```python
from build123d import *

# Parameters (mm, degrees)
SKETCH2_W                                            = 184.15
SKETCH2_H                                            = 190.5
BOSS_EXTRUDE1_DEPTH                                  = 50.8
SHELL1_T                                             = -5.08
CSK_FOR_M6_HEX_SOCKET_COUNTERSUNK_CAP_SC_D           = 6.6
CSK_FOR_M6_HEX_SOCKET_COUNTERSUNK_CAP_SC_DEPTH       = 11.733159957
CSK_FOR_M6_HEX_SOCKET_COUNTERSUNK_CAP_SC_CSINK_D     = 13.44
CSK_FOR_M6_HEX_SOCKET_COUNTERSUNK_CAP_SC_CSINK_ANGLE = 90
CSK_FOR_M6_HEX_SOCKET_COUNTERSUNK_CAP_SC_TIP         = 1.982840043
FILLET1_R                                            = 2.54


with BuildPart() as part:
    # Sketch2 → Boss-Extrude1 (new body)
    with BuildSketch(Plane(origin=(0, 0, 0), x_dir=(1, 0, 0), z_dir=(0, 1, 0))):
        Rectangle(SKETCH2_W, SKETCH2_H)
    extrude(amount=-BOSS_EXTRUDE1_DEPTH)

    # Shell1
    shell1_openings = [part.faces().sort_by_distance(p)[0] for p in [
        (0, -50.8, 0),
    ]]
    offset(amount=SHELL1_T, openings=shell1_openings, kind=Kind.INTERSECTION)

    # Loft1: read off the stored shape, not the designer's step
    # Loft1: loft between two sections, ruled curve by curve
    loft1_from = [
        Edge.make_bspline([(68.241223487, -26.310119776, -101.6), (68.532768976, -26.616911457, -101.6), (68.863871753, -26.909333008, -101.6), (69.601572379, -27.439191099, -101.6), (70.008225028, -27.676441112, -101.6), (70.882099248, -28.069631586, -101.6), (71.349251098, -28.225355381, -101.6), (72.31767022, -28.435607084, -101.6), (72.818735502, -28.489985667, -101.6), (73.821125836, -28.489985667, -101.6), (74.322191118, -28.435607084, -101.6), (75.29061024, -28.225355381, -101.6), (75.757762089, -28.069631586, -101.6), (76.631636309, -27.676441112, -101.6), (77.038288959, -27.439191099, -101.6), (77.775989584, -26.909333008, -101.6), (78.107092362, -26.616911457, -101.6), (78.39863785, -26.310119776, -101.6)], [0, 0, 0, 0, 0.125, 0.125, 0.25, 0.25, 0.375, 0.375, 0.5, 0.5, 0.625, 0.625, 0.75, 0.75, 0.875, 0.875, 1, 1, 1, 1], 3),
        Edge.make_bspline([(78.39863785, -26.310119776, -101.6), (78.675694815, -26.018574288, -101.6), (78.937226358, -25.692808769, -101.6), (79.407739121, -24.977845102, -101.6), (79.616581189, -24.588623733, -101.6), (79.961046476, -23.760489668, -101.6), (80.096520237, -23.321639377, -101.6), (80.279103538, -22.416392759, -101.6), (80.326114413, -21.950142771, -101.6), (80.326114413, -21.017461075, -101.6), (80.279103538, -20.551211086, -101.6), (80.096520237, -19.645964468, -101.6), (79.961046476, -19.207114178, -101.6), (79.616581189, -18.378980112, -101.6), (79.407739121, -17.989758743, -101.6), (78.937226358, -17.274795077, -101.6), (78.675694815, -16.949029558, -101.6), (78.39863785, -16.657484069, -101.6)], [0, 0, 0, 0, 0.125, 0.125, 0.25, 0.25, 0.375, 0.375, 0.5, 0.5, 0.625, 0.625, 0.75, 0.75, 0.875, 0.875, 1, 1, 1, 1], 3),
        Edge.make_bspline([(68.241223487, -16.657484069, -101.6), (67.964166523, -16.949029558, -101.6), (67.70263498, -17.274795077, -101.6), (67.232122217, -17.989758743, -101.6), (67.023280149, -18.378980112, -101.6), (66.678814862, -19.207114178, -101.6), (66.543341101, -19.645964468, -101.6), (66.3607578, -20.551211086, -101.6), (66.313746925, -21.017461075, -101.6), (66.313746925, -21.950142771, -101.6), (66.3607578, -22.416392759, -101.6), (66.543341101, -23.321639377, -101.6), (66.678814862, -23.760489668, -101.6), (67.023280149, -24.588623733, -101.6), (67.232122217, -24.977845102, -101.6), (67.70263498, -25.692808769, -101.6), (67.964166523, -26.018574288, -101.6), (68.241223487, -26.310119776, -101.6)], [0, 0, 0, 0, 0.125, 0.125, 0.25, 0.25, 0.375, 0.375, 0.5, 0.5, 0.625, 0.625, 0.75, 0.75, 0.875, 0.875, 1, 1, 1, 1], 3),
        Edge.make_bspline([(78.39863785, -16.657484069, -101.6), (78.107092362, -16.350692388, -101.6), (77.775989584, -16.058270838, -101.6), (77.038288959, -15.528412746, -101.6), (76.631636309, -15.291162733, -101.6), (75.757762089, -14.89797226, -101.6), (75.29061024, -14.742248464, -101.6), (74.322191118, -14.531996762, -101.6), (73.821125836, -14.477618178, -101.6), (72.818735502, -14.477618178, -101.6), (72.31767022, -14.531996762, -101.6), (71.349251098, -14.742248464, -101.6), (70.882099248, -14.89797226, -101.6), (70.008225028, -15.291162733, -101.6), (69.601572379, -15.528412746, -101.6), (68.863871753, -16.058270838, -101.6), (68.532768976, -16.350692388, -101.6), (68.241223487, -16.657484069, -101.6)], [0, 0, 0, 0, 0.125, 0.125, 0.25, 0.25, 0.375, 0.375, 0.5, 0.5, 0.625, 0.625, 0.75, 0.75, 0.875, 0.875, 1, 1, 1, 1], 3),
    ]
    loft1_to = [
        Edge.make_bspline([(62.059516528, -35.333897225, -95.25), (63.205579438, -35.333897225, -95.25), (64.351642348, -35.333897225, -95.25), (66.643768167, -35.333897225, -95.25), (67.789831077, -35.333897225, -95.25), (70.081956897, -35.333897225, -95.25), (71.228019807, -35.333897225, -95.25), (73.520145626, -35.333897225, -95.25), (74.666208536, -35.333897225, -95.25), (76.958334356, -35.333897225, -95.25), (78.104397266, -35.333897225, -95.25), (80.396523085, -35.333897225, -95.25), (81.542585995, -35.333897225, -95.25), (83.834711815, -35.333897225, -95.25), (84.980774725, -35.333897225, -95.25), (87.272900544, -35.333897225, -95.25), (88.418963454, -35.333897225, -95.25), (89.565026364, -35.333897225, -95.25)], [0, 0, 0, 0, 0.125, 0.125, 0.25, 0.25, 0.375, 0.375, 0.5, 0.5, 0.625, 0.625, 0.75, 0.75, 0.875, 0.875, 1, 1, 1, 1], 3),
        Edge.make_bspline([(89.565026364, -35.333897225, -95.25), (89.565026364, -34.244788582, -95.25), (89.565026364, -33.15567994, -95.25), (89.565026364, -30.977462655, -95.25), (89.565026364, -29.888354013, -95.25), (89.565026364, -27.710136729, -95.25), (89.565026364, -26.621028086, -95.25), (89.565026364, -24.442810802, -95.25), (89.565026364, -23.353702159, -95.25), (89.565026364, -21.175484875, -95.25), (89.565026364, -20.086376233, -95.25), (89.565026364, -17.908158948, -95.25), (89.565026364, -16.819050306, -95.25), (89.565026364, -14.640833021, -95.25), (89.565026364, -13.551724379, -95.25), (89.565026364, -11.373507094, -95.25), (89.565026364, -10.284398452, -95.25), (89.565026364, -9.19528981, -95.25)], [0, 0, 0, 0, 0.125, 0.125, 0.25, 0.25, 0.375, 0.375, 0.5, 0.5, 0.625, 0.625, 0.75, 0.75, 0.875, 0.875, 1, 1, 1, 1], 3),
        Edge.make_bspline([(62.059516528, -9.19528981, -95.25), (62.059516528, -10.284398452, -95.25), (62.059516528, -11.373507094, -95.25), (62.059516528, -13.551724379, -95.25), (62.059516528, -14.640833021, -95.25), (62.059516528, -16.819050306, -95.25), (62.059516528, -17.908158948, -95.25), (62.059516528, -20.086376233, -95.25), (62.059516528, -21.175484875, -95.25), (62.059516528, -23.353702159, -95.25), (62.059516528, -24.442810802, -95.25), (62.059516528, -26.621028086, -95.25), (62.059516528, -27.710136729, -95.25), (62.059516528, -29.888354013, -95.25), (62.059516528, -30.977462655, -95.25), (62.059516528, -33.15567994, -95.25), (62.059516528, -34.244788582, -95.25), (62.059516528, -35.333897225, -95.25)], [0, 0, 0, 0, 0.125, 0.125, 0.25, 0.25, 0.375, 0.375, 0.5, 0.5, 0.625, 0.625, 0.75, 0.75, 0.875, 0.875, 1, 1, 1, 1], 3),
        Edge.make_bspline([(89.565026364, -9.19528981, -95.25), (88.418963454, -9.19528981, -95.25), (87.272900544, -9.19528981, -95.25), (84.980774725, -9.19528981, -95.25), (83.834711815, -9.19528981, -95.25), (81.542585995, -9.19528981, -95.25), (80.396523085, -9.19528981, -95.25), (78.104397266, -9.19528981, -95.25), (76.958334356, -9.19528981, -95.25), (74.666208536, -9.19528981, -95.25), (73.520145626, -9.19528981, -95.25), (71.228019807, -9.19528981, -95.25), (70.081956897, -9.19528981, -95.25), (67.789831077, -9.19528981, -95.25), (66.643768167, -9.19528981, -95.25), (64.351642348, -9.19528981, -95.25), (63.205579438, -9.19528981, -95.25), (62.059516528, -9.19528981, -95.25)], [0, 0, 0, 0, 0.125, 0.125, 0.25, 0.25, 0.375, 0.375, 0.5, 0.5, 0.625, 0.625, 0.75, 0.75, 0.875, 0.875, 1, 1, 1, 1], 3),
    ]
    loft1 = Solid(Shell([*[Face.make_surface_from_curves(loft1_from[k], loft1_to[k]) for k in range(4)], Face(Wire(loft1_from)), Face(Wire(loft1_to))]))
    add(loft1)

    # CSK for M6 Hex Socket Countersunk Cap Screw1
    with Locations(Plane(origin=(0, 0, -101.6), x_dir=(-1, 0, 0), z_dir=(0, 0, -1))):
        with Locations((-73.319930669, -21.483801923)):
            CounterSinkHole(CSK_FOR_M6_HEX_SOCKET_COUNTERSUNK_CAP_SC_D / 2, CSK_FOR_M6_HEX_SOCKET_COUNTERSUNK_CAP_SC_CSINK_D / 2, depth=CSK_FOR_M6_HEX_SOCKET_COUNTERSUNK_CAP_SC_DEPTH, counter_sink_angle=CSK_FOR_M6_HEX_SOCKET_COUNTERSUNK_CAP_SC_CSINK_ANGLE)
            with Locations((0, 0, -(CSK_FOR_M6_HEX_SOCKET_COUNTERSUNK_CAP_SC_DEPTH + CSK_FOR_M6_HEX_SOCKET_COUNTERSUNK_CAP_SC_TIP / 2))):  # 118° drill point
                Cone(0, CSK_FOR_M6_HEX_SOCKET_COUNTERSUNK_CAP_SC_D / 2, CSK_FOR_M6_HEX_SOCKET_COUNTERSUNK_CAP_SC_TIP, mode=Mode.SUBTRACT)

    # Fillet1
    fillet1_edges = [part.edges().sort_by_distance(p)[0] for p in [
        (0, 0, 95.25),
        (-92.075, 0, 0),
        (0, 0, -95.25),
        (92.075, 0, 0),
    ]]
    fillet(fillet1_edges, radius=FILLET1_R)


solid = part.part
```
Model file for the job. Use its own axes, mm. A direction names the side the tool comes from. Give positions to 0.01 mm unless a question says otherwise; leave off trailing zeros. Loops run counter-clockwise (first coordinate to the right, second up) from the corner with the lowest first, then second, coordinate; pieces in that order, holes last. Notation, with made-up numbers: (83, 58) -> (141, 58) arc R38 cw to (141, 96) -> close; hole circle Ø7 at (-36.75, -33.5). An arc over 180 degrees is marked (long way). Write each question's results on one line, items separated by ' | '.
(1) Tool access for faces 4 (the flat face through (-86.995, -28, 1)), 5 (the flat face through (-92.075, -26, 1)): list every direction of +Z, -Z, +X, -X, +Y, -Y with a clear straight run to the whole face (end or side of a thin tool).
Geometry results:
face 4: -Y | face 5: +Z, -Z, -X, +Y, -Y
(2) Cut at A-A on z = 26. List the corners of the cut face in (x, y) (3 decimals).
Geometry results:
outline: (-92.075, -50.8) -> (-86.995, -50.8) -> (-86.995, -5.08) -> (86.995, -5.08) -> (86.995, -50.8) -> (92.075, -50.8) -> (92.075, -2.54) arc R2.54 ccw to (89.535, 0) -> (-89.535, 0) arc R2.54 ccw to (-92.075, -2.54) -> close
(3) Cut at B-B on x = -73. List the corners of the cut face in (y, z), and give its area (3 significant figures).
Geometry results:
outline: (-50.8, -95.25) -> (-2.54, -95.25) arc R2.54 ccw to (0, -92.71) -> (0, 92.71) arc R2.54 ccw to (-2.54, 95.25) -> (-50.8, 95.25) -> (-50.8, 90.17) -> (-5.08, 90.17) -> (-5.08, -90.17) -> (-50.8, -90.17) -> close | area: 1,430 mm²
(4) Pull direction X, two halves, no side cores. Call faces 1 (the flat face through (92.075, -26, 1)), 2 (the flat face through (-1, -26, 95.25)), 3 (the cylindrical face through (76.468, -20.493, -94.119)): released by +X, released by -X, zero draft, split by the parting line, or undercut.
Geometry results:
face 1: released by +X | face 2: zero draft | face 3: undercut
(5) Probe line 1 along Z through (x, y) = (-61.5, -13); line 2 along X through (y, z) = (-6, 28.5) (3 decimals); line 3 along Y through (x, z) = (31, -7). List the from-to ranges inside material, lowest first.
Geometry results:
line 1: z = -95.25 to -90.17, 90.17 to 95.25 | line 2: x = -92.075 to -86.995, 86.995 to 92.075 | line 3: y = -5.08 to 0
(6) Flat gauge pins, fed straight in: pin 1 Ø12 at (x, z) = (-53.5, 63.5) entering from -Y; pin 2 Ø8.5 at (x, y) = (73.32, -21.48) entering from -Z; pin 3 Ø8 at (x, y) = (-64, -35.5) entering from -Z. Where does each tip first touch, or does it go through?
Geometry results:
pin 1: stops at y = -5.08 | pin 2: stops at z = -99.13 | pin 3: stops at z = -95.25
